```python
from build123d import *

# Parameters (mm, degrees)
BASE_EXTRUSION_DEPTH    = 21
ESQUISSE2_W             = 56.002380091
ESQUISSE2_H             = 20.539256902
ENL_V_MAT_EXTRU_1_DEPTH = 78.129760793
ESQUISSE3_R             = 5
ENL_V_MAT_EXTRU_2_DEPTH = 6
ESQUISSE4_R             = 2.75
ENL_V_MAT_EXTRU_3_DEPTH = 6


with BuildPart() as part:
    # Esquisse1 → Base-Extrusion (new body)
    with BuildSketch(Plane.XY):
        with BuildLine():
            Line((0, 0), (0, 10))
            Line((0, 10), (60, 10))
            Line((60, 10), (72, 3.07179677))
            Line((72, 3.07179677), (72, -8))
            Line((72, -8), (70, -8))
            Line((70, -8), (61, 1))
            Line((61, 1), (52, -8))
            Line((52, -8), (50, -8))
            ThreePointArc((50, -8), (46.526596349, -2.254033308), (40.202041029, 0))
            Line((40.202041029, 0), (0, 0))
        make_face()
    extrude(amount=BASE_EXTRUSION_DEPTH)

    # Esquisse2 → Enlèv. mat.-Extru.1 (cut, through all)
    with BuildSketch(Plane(origin=(0, 10, 0), x_dir=(-1, 0, 0), z_dir=(0, 1, 0))):
        with Locations((-66.001190046, 15.769628451)):
            Rectangle(ESQUISSE2_W, ESQUISSE2_H)
    extrude(amount=-ENL_V_MAT_EXTRU_1_DEPTH, mode=Mode.SUBTRACT)

    # Esquisse3 → Enlèv. mat.-Extru.2 (cut)
    with BuildSketch(Plane.XZ):
        with Locations(Location((28, 15.5, 0), (0, 0, 270))):
            Circle(ESQUISSE3_R)
        with Locations(Location((10, 15.5, 0), (0, 0, 270))):
            Circle(ESQUISSE3_R)
    extrude(amount=-ENL_V_MAT_EXTRU_2_DEPTH, mode=Mode.SUBTRACT)

    # Esquisse4 → Enlèv. mat.-Extru.3 (cut)
    with BuildSketch(Plane.XZ.offset(-6)):
        with Locations(Location((28, 15.5, 0), (0, 0, 270))):
            Circle(ESQUISSE4_R)
        with Locations(Location((10, 15.5, 0), (0, 0, 270))):
            Circle(ESQUISSE4_R)
    extrude(amount=-ENL_V_MAT_EXTRU_3_DEPTH, mode=Mode.SUBTRACT)


solid = part.part
```
Can you work these out from the model? Positions are in its coordinate system, mm. A direction names the side the tool comes from. Coordinates: 2 decimals unless noted, no trailing zeros. Loops run counter-clockwise (first coordinate to the right, second up) from the corner with the lowest first, then second, coordinate; pieces in that order, holes last. Notation, with made-up numbers: (59, 3) - (76, 3) arc R21 ccw to (76, 10) - close; hole circle Ø9 at (27, 51). An arc over 180 degrees is marked (long way). Use a Markdown table: item, result.
Item 1: Will these pins go through, and if not, where does the flat tip stop? pin 1 (10 mm diameter, centred on y = 4, z = 5.5, fed in from +X); pin 2 (10 mm diameter, centred on y = -2, z = 12, fed in from +X); pin 3 (5 mm diameter, centred on x = 26.5, z = 15, fed in from -Y); pin 4 (1.5 mm diameter, centred on x = 34.5, y = -2.5, fed in from +Z).
Numbers:
| item | result |
|---|---|
| pin 1 | stops at x = 72 |
| pin 2 | stops at x = 38 |
| pin 3 | stops at y = 6 |
| pin 4 | passes through |
Item 2: If I drill on probe 1 along X at (y, z) = (1.6, 15.5); probe 2 along X at (y, z) = (7.95, 15.5); probe 3 along Z at (x, y) = (68, 4.25), over which ranges is the centre line in solid material (lowest first)? Write a range as from..to.
Numbers:
| item | result |
|---|---|
| probe 1 | x = 0..5, 15..23, 33..38 |
| probe 2 | x = 0..7.25, 12.75..25.25, 30.75..38 |
| probe 3 | z = 0..5.5 |
Item 3: I want a section at B-B on z = 15.5. Please give me the cut outline in (x, y).
Numbers:
| item | result |
|---|---|
| outline | (0, 0) - (5, 0) - (5, 6) - (7.25, 6) - (7.25, 10) - (0, 10) - close; (12.75, 6) - (15, 6) - (15, 0) - (23, 0) - (23, 6) - (25.25, 6) - (25.25, 10) - (12.75, 10) - close; (30.75, 6) - (33, 6) - (33, 0) - (38, 0) - (38, 10) - (30.75, 10) - close |
Item 4: I want a section at C-C on y = -3. Please give me the cut outline in (x, z), and give its area (3 significant figures).
Numbers:
| item | result |
|---|---|
| outline | (47.34, 0) - (57, 0) - (57, 5.5) - (47.34, 5.5) - close; (65, 0) - (72, 0) - (72, 5.5) - (65, 5.5) - close |
| area | 91.6 mm2 |
Item 5: We'd pull the mould along X, two halves only. Please class faces 5 (the face through (11.859, 7.972, 17.527)), 6 (the face through (46.601, -2.315, 2.712)), 7 (the face through (37, 3, 0)), 8 (the face through (38, 5, 13)): released by +X, released by -X, zero draft, split by the parting line, or undercut.
Numbers:
| item | result |
|---|---|
| face 5 | undercut |
| face 6 | released by -X |
| face 7 | zero draft |
| face 8 | released by +X |
Item 6: I want a section at D-D on z = 4. Please give me the cut outline in (x, y).
Numbers:
| item | result |
|---|---|
| outline | (0, 0) - (40.2, 0) arc R10 cw to (50, -8) - (52, -8) - (61, 1) - (70, -8) - (72, -8) - (72, 3.07) - (60, 10) - (0, 10) - close |
Item 7: For faces 1 (the face through (66, -4, 3)), 2 (the face through (23.12, 2.96, 16.58)), 3 (the face through (72, -2, 3)), 4 (the face through (20, 0, 8)), which set-ups out of +Z, -Z, +X, -X, +Y, -Y let a thin tool reach every point of the face, with its end or its side?
Numbers:
| item | result |
|---|---|
| face 1 | +Z, -Z, -Y |
| face 2 | -Y |
| face 3 | +Z, -Z, +X, +Y, -Y |
| face 4 | +Z, -Z, -X, -Y |
Item 8: I want a section at A-A on x = 10. Please give me the cut outline in (y, z).
Numbers:
| item | result |
|---|---|
| outline | (0, 0) - (10, 0) - (10, 12.75) - (6, 12.75) - (6, 10.5) - (0, 10.5) - close; (0, 20.5) - (6, 20.5) - (6, 18.25) - (10, 18.25) - (10, 21) - (0, 21) - close |
